```python
from build123d import *

# Parameters (mm, degrees)
SKETCH021_W          = 58.2
SKETCH021_H          = 55.7
SKETCH021_R          = 1.75
PAD007_DEPTH         = 1.6
SKETCH028_W          = 53.7
SKETCH028_H          = 55.7
SKETCH028_W_2        = 50.5
SKETCH028_H_2        = 52.5
PAD008_DEPTH         = 40
FILLET003_R          = 1
SKETCH026_W          = 6.2
SKETCH026_H          = 4
SKETCH026_W_2        = 5
POCKET005_DEPTH      = 27.851
POCKET005_DEPTH_BACK = 27.851
SKETCH023_W          = 9
SKETCH023_H          = 3.8
POCKET006_DEPTH      = 31.351
SKETCH062_W          = 9
SKETCH062_H          = 3.8
POCKET021_DEPTH      = 26.851
SKETCH024_R          = 3.2
PAD006_DEPTH         = 3
SKETCH038_R          = 1.75
POCKET010_DEPTH      = 4.601


with BuildPart() as part:
    # Sketch021 → Pad007 (new body)
    with BuildSketch(Plane.XY):
        with Locations((-2.25, 0)):
            Rectangle(SKETCH021_W, SKETCH021_H)
        with Locations((19.652, 0)):
            Circle(SKETCH021_R, mode=Mode.SUBTRACT)
    extrude(amount=PAD007_DEPTH)

    # Sketch028 → Pad008 (join)
    with BuildSketch(Plane.XY.offset(1.6)):
        Rectangle(SKETCH028_W, SKETCH028_H)
        Rectangle(SKETCH028_W_2, SKETCH028_H_2, mode=Mode.SUBTRACT)
    extrude(amount=PAD008_DEPTH)

    # Fillet003
    fillet003_edges = [part.edges().sort_by_distance(p)[0] for p in [
        (-31.35, -27.85, 0.8),
        (-26.85, 27.85, 21.6),
        (-25.25, 26.25, 21.6),
        (26.85, 27.85, 20.8),
        (25.25, 26.25, 21.6),
        (26.85, -27.85, 20.8),
        (25.25, -26.25, 21.6),
        (-26.85, -27.85, 21.6),
        (-25.25, -26.25, 21.6),
        (-31.35, 27.85, 0.8),
    ]]
    fillet(fillet003_edges, radius=FILLET003_R)

    # Sketch026 → Pocket005 (cut, two sides)
    with BuildSketch(Plane.XZ) as pocket005_sk:
        with Locations((0, 35.8)):
            Rectangle(SKETCH026_W, SKETCH026_H)
        with Locations((-18, 35.8)):
            Rectangle(SKETCH026_W_2, SKETCH026_H)
        with Locations((18, 35.8)):
            Rectangle(SKETCH026_W_2, SKETCH026_H)
        with BuildLine():
            Line((22.5, 41.6), (23.5, 41.6))
            Line((23.5, 41.6), (23.5, 26.6))
            ThreePointArc((22.5, 27.6), (22.792893, 26.892893), (23.5, 26.6))
            Line((22.5, 27.6), (22.5, 41.6))
        make_face()
        with BuildLine():
            Line((-23.5, 41.6), (-22.5, 41.6))
            Line((-22.5, 41.6), (-22.5, 27.6))
            ThreePointArc((-23.5, 26.6), (-22.792893, 26.892893), (-22.5, 27.6))
            Line((-23.5, 26.6), (-23.5, 41.6))
        make_face()
    extrude(amount=-POCKET005_DEPTH, mode=Mode.SUBTRACT)
    extrude(pocket005_sk.sketch, amount=POCKET005_DEPTH_BACK, mode=Mode.SUBTRACT)

    # Sketch023 → Pocket006 (cut, through all)
    with BuildSketch(Plane.YZ):
        with Locations((-16, 39.7)):
            Rectangle(SKETCH023_W, SKETCH023_H)
        with Locations((16, 39.7)):
            Rectangle(SKETCH023_W, SKETCH023_H)
        with BuildLine():
            Line((-18.733, 22.8), (18.733, 22.8))
            ThreePointArc((23.733, 17.8), (22.268534, 21.335534), (18.733, 22.8))
            Line((23.733, 1.6), (23.733, 17.8))
            Line((-23.733, 1.6), (23.733, 1.6))
            Line((-23.733, 17.8), (-23.733, 1.6))
            ThreePointArc((-18.733, 22.8), (-22.268534, 21.335534), (-23.733, 17.8))
        make_face()
    extrude(amount=-POCKET006_DEPTH, mode=Mode.SUBTRACT)

    # Sketch062 → Pocket021 (cut, through all)
    with BuildSketch(Plane.YZ):
        with Locations((-16, 39.7)):
            Rectangle(SKETCH062_W, SKETCH062_H)
        with Locations((16, 39.7)):
            Rectangle(SKETCH062_W, SKETCH062_H)
        with BuildLine():
            Line((-23.733, 17.6), (-23.733, 10.6))
            ThreePointArc((-23.733, 10.6), (-23.440107, 9.892893), (-22.733, 9.6))
            Line((-22.733, 9.6), (-15.733, 9.6))
            ThreePointArc((-15.733, 9.6), (-15.025893, 9.892893), (-14.733, 10.6))
            Line((-14.733, 17.6), (-14.733, 10.6))
            ThreePointArc((-14.733, 17.6), (-15.025893, 18.307107), (-15.733, 18.6))
            Line((-22.733, 18.6), (-15.733, 18.6))
            ThreePointArc((-22.733, 18.6), (-23.440107, 18.307107), (-23.733, 17.6))
        make_face()
        with BuildLine():
            Line((22.733, 9.6), (15.733, 9.6))
            ThreePointArc((14.733, 10.6), (15.025893, 9.892893), (15.733, 9.6))
            Line((14.733, 10.6), (14.733, 17.6))
            ThreePointArc((15.733, 18.6), (15.025893, 18.307107), (14.733, 17.6))
            Line((15.733, 18.6), (22.733, 18.6))
            ThreePointArc((23.733, 17.6), (23.440107, 18.307107), (22.733, 18.6))
            Line((23.733, 10.6), (23.733, 17.6))
            ThreePointArc((22.733, 9.6), (23.440107, 9.892893), (23.733, 10.6))
        make_face()
    extrude(amount=POCKET021_DEPTH, mode=Mode.SUBTRACT)

    # Sketch024 → Pad006 (join)
    with BuildSketch(Plane.XY.offset(1.6)):
        with Locations((-15.348, 15.621)):
            Circle(SKETCH024_R)
        with Locations((-28.048, -19.431)):
            Circle(SKETCH024_R)
        with Locations((-15.348, -19.431)):
            Circle(SKETCH024_R)
        with Locations((-28.048, 15.621)):
            Circle(SKETCH024_R)
    extrude(amount=PAD006_DEPTH)

    # Sketch038 → Pocket010 (cut, through all)
    with BuildSketch(Plane.XY.offset(4.6)):
        with Locations((-28.048, 15.621)):
            Circle(SKETCH038_R)
        with Locations((-15.348, 15.621)):
            Circle(SKETCH038_R)
        with Locations((-15.348, -19.431)):
            Circle(SKETCH038_R)
        with Locations((-28.048, -19.431)):
            Circle(SKETCH038_R)
    extrude(amount=-POCKET010_DEPTH, mode=Mode.SUBTRACT)


solid = part.part
```
Geometry: final body of the model. Coordinates: model frame, mm. A direction names the side the tool comes from. Coordinates: 2 decimals unless noted, no trailing zeros. Order: outer loops, then holes, each group sorted by start corner. A loop starts at its lowest first (then second) coordinate and runs counter-clockwise, first axis right, second up. Notation, with made-up numbers: (-3.5, 16) -> (13.5, 16) arc R18 ccw to (13.5, 43) -> close; hole circle Ø7 at (7, 68). An arc over 180 degrees is marked (long way). Use CSV: the item, a comma, the result in double quotes.
1) Section C-C on y = -1. Output: boundary loops of the cut face in (x, z), then the cut area to 3 significant figures.
Findings:
outline,"(-31.35, 0) -> (18.22, 0) -> (18.22, 1.6) -> (-31.35, 1.6) -> close; (-26.85, 22.8) -> (-25.25, 22.8) -> (-25.25, 41.6) -> (-26.85, 41.6) -> close; (21.09, 0) -> (26.85, 0) -> (26.85, 41.6) -> (25.25, 41.6) -> (25.25, 1.6) -> (21.09, 1.6) -> close"
area,"183 mm^2"
2) Line query: line 1 (X direction, y = 22, z = 28); line 2 (Y direction, x = -12, z = 30); line 3 (Z direction, x = -26.5, y = -2). Output: solid intervals per line, ascending.
Findings:
line 1,"x = -26.85 to -25.25, 25.25 to 26.85"
line 2,"y = -27.85 to -26.25, 26.25 to 27.85"
line 3,"z = 0 to 1.6, 22.8 to 41.6"
3) Access query for faces 4 (the flat face through (26, -23.733, 14)), 5 (the flat face through (-18, -27, 33.8)), 6 (the flat face through (-26, -20.5, 40)). Directions: +Z, -Z, +X, -X, +Y, -Y. A direction counts if a zero-diameter tool reaches every point of the face in a straight line with its end or side. Return the directions, or none.
Findings:
face 4,"+X, -X"
face 5,"+Y, -Y"
face 6,"+Z, +X, -X"
4) Section A-A on y = 5. Output: boundary loops of the cut face in (x, z).
Findings:
outline,"(-31.35, 0) -> (26.85, 0) -> (26.85, 41.6) -> (25.25, 41.6) -> (25.25, 1.6) -> (-31.35, 1.6) -> close; (-26.85, 22.8) -> (-25.25, 22.8) -> (-25.25, 41.6) -> (-26.85, 41.6) -> close"
5) Pin query (flat end, axial travel): pin 1 Ø3 at (x, y) = (-14.5, -19.5) entering from +Z; pin 2 Ø4 at (x, y) = (16.5, -20.5) entering from +Z; pin 3 Ø1.9 at (x, y) = (-15.5, 15) entering from +Z; pin 4 Ø3 at (x, y) = (-28.048, -19.431) entering from +Z. Return the tip coordinate at first contact, or that it passes through.
Findings:
pin 1,"stops at z = 4.6"
pin 2,"stops at z = 1.6"
pin 3,"passes through"
pin 4,"stops at z = 37.8"
6) Section B-B on z = 5.5. Output: boundary loops of the cut face in (x, y), then the cut area to 3 significant figures.
Findings:
outline,"(-26.85, -26.85) arc R1 ccw to (-25.85, -27.85) -> (25.85, -27.85) arc R1 ccw to (26.85, -26.85) -> (26.85, 26.85) arc R1 ccw to (25.85, 27.85) -> (-25.85, 27.85) arc R1 ccw to (-26.85, 26.85) -> (-26.85, 23.73) -> (-25.25, 23.73) -> (-25.25, 25.25) arc R1 cw to (-24.25, 26.25) -> (24.25, 26.25) arc R1 cw to (25.25, 25.25) -> (25.25, -25.25) arc R1 cw to (24.25, -26.25) -> (-24.25, -26.25) arc R1 cw to (-25.25, -25.25) -> (-25.25, -23.73) -> (-26.85, -23.73) -> close"
area,"264 mm^2"
7) Section D-D on x = 13. Output: boundary loops of the cut face in (y, z), then the cut area to 3 significant figures.
Findings:
outline,"(-27.85, 0) -> (27.85, 0) -> (27.85, 41.6) -> (26.25, 41.6) -> (26.25, 1.6) -> (-26.25, 1.6) -> (-26.25, 41.6) -> (-27.85, 41.6) -> close"
area,"217 mm^2"
8) Mould query, pull axis Z, two halves, no side actions, for faces 1 (the flat face through (-26, 25, 41.6)), 2 (the flat face through (-3, -27.85, 21)), 3 (the flat face through (20.5, 27, 36)). Classes: +Z half, -Z half, draft (parallel to the pull), parting line (faces both ways), or undercut.
Findings:
face 1,"+Z half"
face 2,"draft"
face 3,"undercut"
